Autodesk Inventor part; units mm, degrees
ref_plane "YZ Plane" through (0, 0, 0) normal (1, 0, 0) x (0, 1, 0)
ref_plane "XZ Plane" through (0, 0, 0) normal (0, 1, 0) x (-1, 0, 0)
ref_plane "XY Plane" through (0, 0, 0) normal (0, 0, 1) x (1, 0, 0)
sketch "スケッチ1" plane through (0, 0, 0) normal (0, 0, 1) x (1, 0, 0)
  line L0 (7.5, 15) -> (-7.5, 15)
  line L1 (-7.5, 15) -> (-7.5, -15)
  line L2 (-7.5, -15) -> (7.5, -15)
  line L3 (7.5, -15) -> (7.5, 15)
  line L4 (7.5, 15) -> (-7.5, -15) construction
  line L5 (-7.5, 15) -> (7.5, -15) construction
  line L6 (-5.5, 13) -> (5.5, 13)
  line L7 (5.5, 13) -> (5.5, -13)
  line L8 (5.5, -13) -> (-5.5, -13)
  line L9 (-5.5, -13) -> (-5.5, 13)
  point P0 (0, 0)
  dimension "d2" = 15
  dimension "d3" = 30
  dimension "d4" = 2
extrude "押し出し1" add sketch "スケッチ1" along normal blind 167
sketch "スケッチ2" plane through (7.5, -15, 0) normal (1, 0, 0) x (0, 0, -1)
  circle A0 centre (-15, 22.5) radius 1.6
  circle A1 centre (-15, 7.5) radius 1.6
  circle A2 centre (-154, 22.5) radius 1.6
  circle A3 centre (-154, 7.5) radius 1.6
  line L0 (0, 30) -> (-167, 30)
  point P0 (0, 15)
  dimension "d7" = 3.2
  dimension "d8" = 3.2
  dimension "d9" = 3.2
  dimension "d10" = 3.2
  dimension "d11" = 15
  dimension "d12" = 15
  dimension "d13" = 7.5
  dimension "d14" = 139
extrude "押し出し2" cut sketch "スケッチ2" against normal through all
sketch "スケッチ4" plane through (-7.5, 15, 0) normal (0, 1, 0) x (1, 0, 0)
  circle A0 centre (7.5, -10) radius 1.6
  circle A1 centre (7.5, -25) radius 1.6
  line L0 (15, 0) -> (0, 0)
  point P0 (7.5, 0)
  point P1 (7.5, 0)
  dimension "d17" = 3.2
  dimension "d18" = 3.2
  dimension "d19" = 15
  dimension "d20" = 10
extrude "押し出し3" cut sketch "スケッチ4" against normal through all
properties part number "オムニ_角柱6" material "アルミニウム 6061"
Check sheet for the modelled part. Datum: model origin and axes. Units: mm. A direction names the side the tool comes from. Give positions to 0.01 mm unless a question says otherwise; leave off trailing zeros. Write each loop counter-clockwise with the first axis right and the second up, starting at its lowest first coordinate (ties: lowest second). Pieces come first, ordered by that corner, then holes. Notation, with made-up numbers: (42, 3) - (69, 3) arc R22 ccw to (69, 33) - close; hole circle Ø10 at (85.5, 60). An arc over 180 degrees is marked (long way). Answer as a JSON object with one key per item and string values. Group by question number.
1) Thickness scan on probe 1 along Z at (x, y) = (0, -14.35); probe 2 along X at (y, z) = (5, 24.5); probe 3 along X at (y, z) = (-14.4, 25). Record the ranges inside material, lowest first. Write a range as from..to.
2) Access from +Z, -Z, +X, -X, +Y, -Y to the whole of each face (thin tool, end or side, straight path). Record for faces 1 (the face through (0, 13, 82)), 2 (the face through (0, -15, 82)).
3) Sectioned sample at B-B (z = 154). Record the cut outline in (x, y), then the cut area to 3 significant figures.
4) Release check for a two-part mould opening along X. For faces 3 (the face through (-7.5, 0, 82)), 4 (the face through (-5.5, 0, 82)), 5 (the face through (-7, 0, 0)) record: pulls with the +X half, pulls with the -X half, needs draft (parallel to the pull), parting line crosses it, or undercut.
5) Sectioned sample at D-D (z = 25). Record the cut outline in (x, y).
6) Sectioned sample at A-A (y = 7.5). Record the cut outline in (x, z), then the cut area to 3 significant figures.
7) Sectioned sample at C-C (y = -3). Record the cut outline in (x, z), then the cut area to 3 significant figures.
Geometry results:
{
 "1": {"probe 1": "z = 0..8.4, 11.6..23.4, 26.6..167", "probe 2": "x = -7.5..-5.5, 5.5..7.5", "probe 3": "x = -7.5..-1.6, 1.6..7.5"},
 "2": {"face 1": "+Z, -Z", "face 2": "+Z, -Z, +X, -X, -Y"},
 "3": {"outline": "(-7.5, -15) - (7.5, -15) - (7.5, -9.1) - (5.5, -9.1) - (5.5, -13) - (-5.5, -13) - (-5.5, -9.1) - (-7.5, -9.1) - close; (-7.5, -5.9) - (-5.5, -5.9) - (-5.5, 5.9) - (-7.5, 5.9) - close; (-7.5, 9.1) - (-5.5, 9.1) - (-5.5, 13) - (5.5, 13) - (5.5, 9.1) - (7.5, 9.1) - (7.5, 15) - (-7.5, 15) - close; (5.5, -5.9) - (7.5, -5.9) - (7.5, 5.9) - (5.5, 5.9) - close", "area": "138 mm^2"},
 "4": {"face 3": "pulls with the -X half", "face 4": "undercut", "face 5": "needs draft"},
 "5": {"outline": "(-7.5, -15) - (-1.6, -15) - (-1.6, -13) - (-5.5, -13) - (-5.5, 13) - (-1.6, 13) - (-1.6, 15) - (-7.5, 15) - close; (1.6, -15) - (7.5, -15) - (7.5, 15) - (1.6, 15) - (1.6, 13) - (5.5, 13) - (5.5, -13) - (1.6, -13) - close"},
 "6": {"outline": "(-7.5, 0) - (-5.5, 0) - (-5.5, 13.4) - (-7.5, 13.4) - close; (-7.5, 16.6) - (-5.5, 16.6) - (-5.5, 152.4) - (-7.5, 152.4) - close; (-7.5, 155.6) - (-5.5, 155.6) - (-5.5, 167) - (-7.5, 167) - close; (5.5, 0) - (7.5, 0) - (7.5, 13.4) - (5.5, 13.4) - close; (5.5, 16.6) - (7.5, 16.6) - (7.5, 152.4) - (5.5, 152.4) - close; (5.5, 155.6) - (7.5, 155.6) - (7.5, 167) - (5.5, 167) - close", "area": "642 mm^2"},
 "7": {"outline": "(-7.5, 0) - (-5.5, 0) - (-5.5, 167) - (-7.5, 167) - close; (5.5, 0) - (7.5, 0) - (7.5, 167) - (5.5, 167) - close", "area": "668 mm^2"}
}
